Job drawing, mm, ordinate dimensions from the low corner. One solid piece. Round coordinates to 2 decimals unless told otherwise and drop trailing zeros. Write each loop counter-clockwise with the first axis right and the second up, starting at its lowest first coordinate (ties: lowest second). Pieces come first, ordered by that corner, then holes.
1) Flat gauge pins, fed straight in: pin 1 (5 mm diameter, centred on y = 22, z = 3.5, fed in from +X); pin 2 (5 mm diameter, centred on y = 85.5, z = 5.5, fed in from -X); pin 3 (3 mm diameter, centred on x = 68.5, z = 6.5, fed in from -Y). Where does each tip first touch, or does it go through?
2) Saw through at A-A (z = 5). Write the cut outline in (x, y).
3) Saw through at B-B (y = 114). Write the cut outline in (x, z), plus the area to 3 significant figures.
4) Wall check: probe 1 along X at (y, z) = (47.5, 1.75); probe 2 along Y at (x, z) = (19, 5.75); probe 3 along Y at (x, z) = (82, 3). Give the ranges that are in metal, low to high.
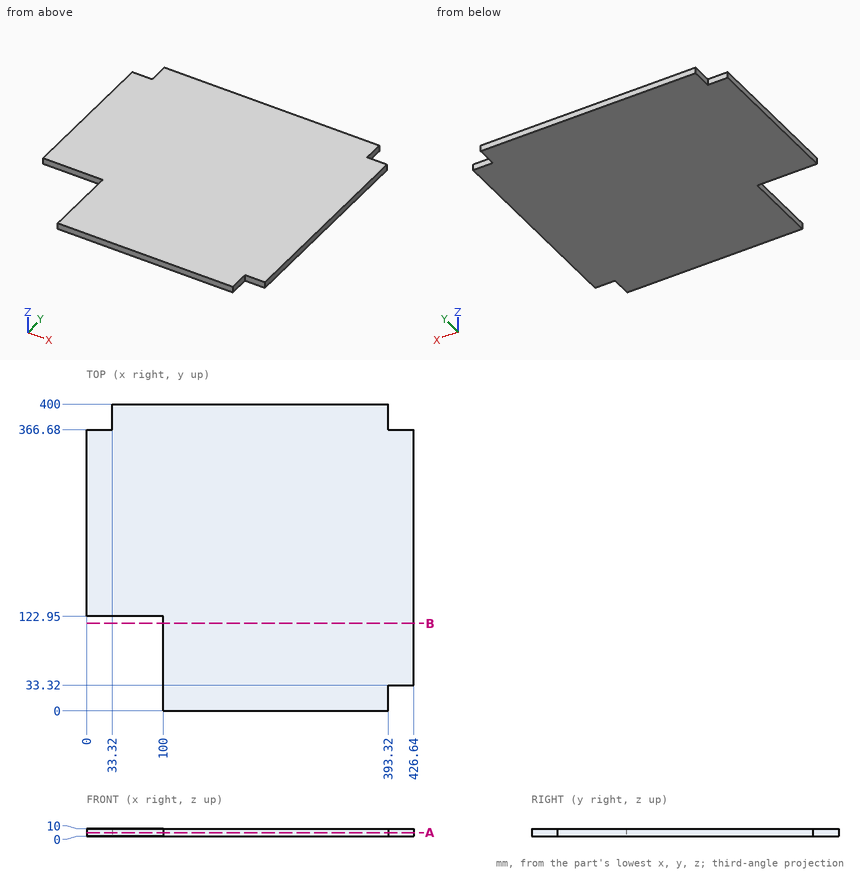
Evaluation:
1. pin 1: stops at x = 393.32
1. pin 2: stops at x = 100
1. pin 3: stops at y = 122.95
2. outline: (0, 122.95) - (100, 122.95) - (100, 0) - (393.32, 0) - (393.32, 33.32) - (426.64, 33.32) - (426.64, 366.68) - (393.32, 366.68) - (393.32, 400) - (33.32, 400) - (33.32, 366.68) - (0, 366.68) - close
3. outline: (100, 0) - (426.64, 0) - (426.64, 10) - (100, 10) - close
3. area: 3,270 mm2
4. probe 1: x = 100 to 426.64
4. probe 2: y = 122.95 to 366.68
4. probe 3: y = 122.95 to 400
